Check sheet for the drawn part. Datum: minimum x, y, z corner. Units: mm. A direction names the side the tool comes from. Coordinates: 2 decimals unless noted, no trailing zeros. Write each loop counter-clockwise with the first axis right and the second up, starting at its lowest first coordinate (ties: lowest second). Pieces come first, ordered by that corner, then holes. Notation, with made-up numbers: (57.25, -26.75) -> (66.25, -26.75) arc R13 ccw to (66.25, -5.75) -> close; hole circle Ø10 at (32.25, 53.25). An arc over 180 degrees is marked (long way). Answer in a Markdown table with one row per item. Add a question column.
1. Cross-section at C-C on y = 41. Record the cut outline in (x, z), and give its area (4 significant figures).
2. Mould release check, pull along X, two halves, no side actions. Record for the marked faces 1, 2 and 3: pulls with the +X half, pulls with the -X half, needs draft (parallel to the pull), parting line crosses it, or undercut.
3. Depth check by flat-ended pin: P1, Ø2, axis at y = 41, z = 5, coming from the +X side; P2, Ø3, axis at x = 11, y = 7, coming from the +Z side; P3, Ø12, axis at x = 14.5, y = 28, coming from the -Z side. Enter the tip coordinate at first touch or a pass-through.
4. Scan lines: L1, parallel to Y at x = 12.5, z = 7.15; L2, parallel to Y at x = 12.5, z = 1.3; L3, parallel to Y at x = 21.5, z = 5.25. Record each from-to range of solid material in increasing order. Write a range as from..to.
5. Set-up check for the marked faces 4, 5 and 6: record each of +Z, -Z, +X, -X, +Y, -Y from which the full face is reachable in a straight line by a thin tool's end or side.
6. Cross-section at A-A on x = 12.5. Give the number of separate pieces and of enclosed holes in the cut face, and give its area (3 significant figures).
7. Cross-section at D-D on x = 4.5. Record the cut outline in (y, z), and give its area (3 significant figures).
8. Cross-section at B-B on z = 4. Record the cut outline in (x, y), and give its area (3 significant figures).
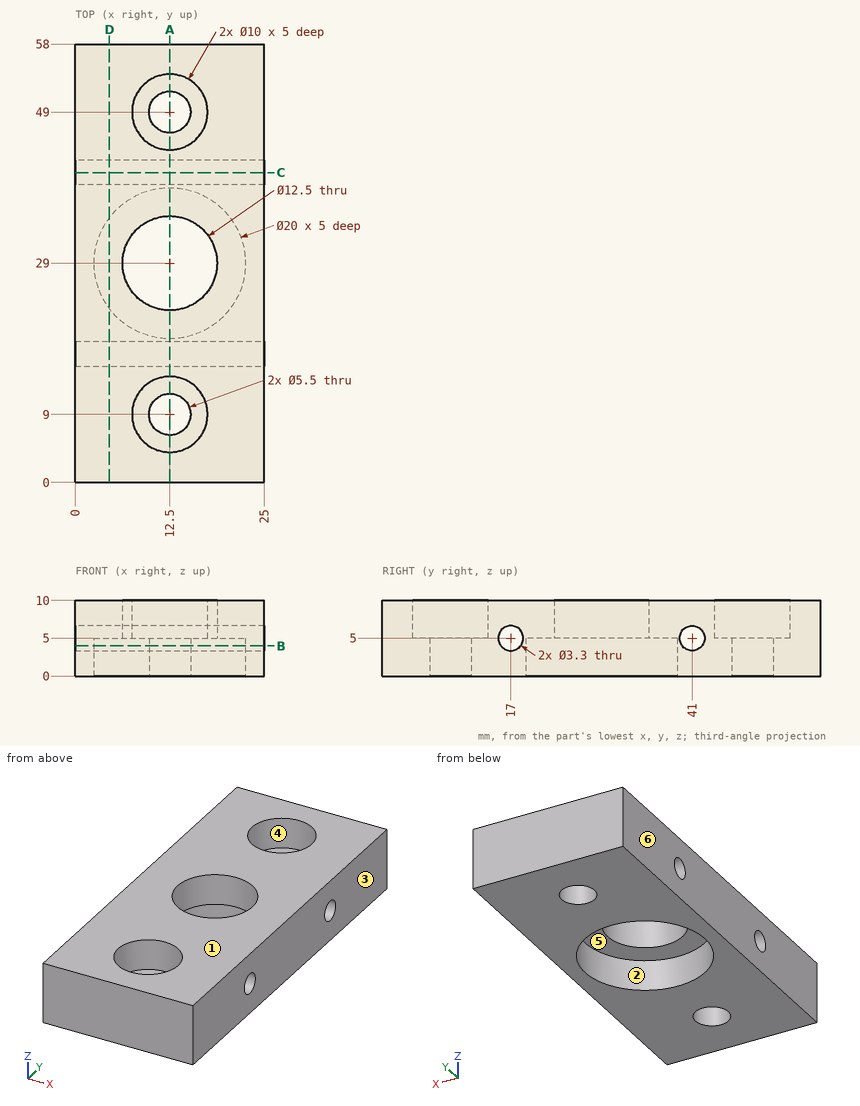
Results found:
| question | item | result |
|---|---|---|
| 1 | outline | (0, 0) -> (25, 0) -> (25, 3.35) -> (0, 3.35) -> close; (0, 6.65) -> (25, 6.65) -> (25, 10) -> (0, 10) -> close |
| 1 | area | 167.5 mm^2 |
| 2 | face 1 | needs draft |
| 2 | face 2 | undercut |
| 2 | face 3 | pulls with the +X half |
| 3 | P1 | passes through |
| 3 | P2 | stops at z = 5 |
| 3 | P3 | stops at z = 5 |
| 4 | L1 | y = 0..4, 14..22.75, 35.25..44, 54..58 |
| 4 | L2 | y = 0..6.25, 11.75..19, 39..46.25, 51.75..58 |
| 4 | L3 | y = 0..15.37, 18.63..39.37, 42.63..58 |
| 5 | face 4 | +Z |
| 5 | face 5 | -Z |
| 5 | face 6 | +Z, -Z, -X, +Y, -Y |
| 6 | separate pieces | 4 |
| 6 | enclosed holes | 2 |
| 6 | area | 245 mm^2 |
| 7 | outline | (0, 0) -> (23, 0) -> (23, 5) -> (35, 5) -> (35, 0) -> (58, 0) -> (58, 10) -> (0, 10) -> close; hole circle Ø3.3 at (17, 5); hole circle Ø3.3 at (41, 5) |
| 7 | area | 503 mm^2 |
| 8 | outline | (0, 0) -> (25, 0) -> (25, 15.69) -> (0, 15.69) -> close; (0, 18.31) -> (25, 18.31) -> (25, 39.69) -> (0, 39.69) -> close; (0, 42.31) -> (25, 42.31) -> (25, 58) -> (0, 58) -> close; hole circle Ø20 at (12.5, 29); hole circle Ø5.5 at (12.5, 9); hole circle Ø5.5 at (12.5, 49) |
| 8 | area | 957 mm^2 |
